```python
from build123d import *

# Parameters (mm, degrees)
SKETCH_1_W          = 99
SKETCH_1_H          = 40
EXTRUDE_1_DEPTH     = 4
SKETCH_2_R          = 2.025
CUT_EXTRUDE_1_DEPTH = 4
FILLET_1_R          = 3
CUT_EXTRUDE_2_DEPTH = 4
FILLET_2_R          = 1
SKETCH_4_R          = 7.5
CUT_EXTRUDE_3_DEPTH = 4
SKETCH_5_W          = 8
SKETCH_5_H          = 27
EXTRUDE_2_DEPTH     = 4
SKETCH_6_R          = 2.025
CUT_EXTRUDE_4_DEPTH = 4
FILLET_3_R          = 1


with BuildPart() as part:
    # 草图1 → 凸台-拉伸1 (new body)
    with BuildSketch(Plane(origin=(0, 0, 0), x_dir=(1, 0, 0), z_dir=(0, 1, 0))):
        Rectangle(SKETCH_1_W, SKETCH_1_H)
    extrude(amount=EXTRUDE_1_DEPTH)

    # 草图2 → 切除-拉伸1 (cut)
    with BuildSketch(Plane(origin=(0, 4, 0), x_dir=(1, 0, 0), z_dir=(0, 1, 0))):
        with Locations((-43.5, 15)):
            Circle(SKETCH_2_R)
        with Locations((-43.5, -15)):
            Circle(SKETCH_2_R)
        with Locations((-25.5, -15)):
            Circle(SKETCH_2_R)
        with Locations((-25.5, 15)):
            Circle(SKETCH_2_R)
    cut_extrude_1 = extrude(amount=-CUT_EXTRUDE_1_DEPTH, mode=Mode.SUBTRACT)

    # 镜向1: 切除-拉伸1 across plane
    add(cut_extrude_1.mirror(Plane(origin=(0, 0, 0), x_dir=(0, 0, 1), z_dir=(1, 0, 0))), mode=Mode.SUBTRACT)

    # 圆角1
    fillet_1_edges = [part.edges().sort_by_distance(p)[0] for p in [
        (49.5, 2, 20),
        (-49.5, 2, 20),
        (-49.5, 2, -20),
        (49.5, 2, -20),
    ]]
    fillet(fillet_1_edges, radius=FILLET_1_R)

    # 草图3 → 切除-拉伸2 (cut)
    with BuildSketch(Plane(origin=(0, 4, 0), x_dir=(1, 0, 0), z_dir=(0, 1, 0))):
        Polygon((-15.333333333, 13.5), (15.333333333, 13.5), (0, 2), align=None)
        Polygon((-21.5, 13.125), (-21.5, -13.125), (-4, 0), align=None)
        Polygon((-15.333333333, -13.5), (15.333333333, -13.5), (0, -2), align=None)
        Polygon((21.5, 13.125), (21.5, -13.125), (4, 0), align=None)
    extrude(amount=-CUT_EXTRUDE_2_DEPTH, mode=Mode.SUBTRACT)

    # 圆角2
    fillet_2_edges = [part.edges().sort_by_distance(p)[0] for p in [
        (15.333333333, 2, -13.5),
        (-15.333333333, 2, -13.5),
        (0, 2, -2),
        (15.333333333, 2, 13.5),
        (0, 2, 2),
        (-15.333333333, 2, 13.5),
        (-21.5, 2, 13.125),
        (-4, 2, 0),
        (-21.5, 2, -13.125),
        (21.5, 2, 13.125),
        (21.5, 2, -13.125),
        (4, 2, 0),
    ]]
    fillet(fillet_2_edges, radius=FILLET_2_R)

    # 草图4 → 切除-拉伸3 (cut)
    with BuildSketch(Plane(origin=(0, 4, 0), x_dir=(1, 0, 0), z_dir=(0, 1, 0))):
        with Locations((-34.5, 0)):
            Circle(SKETCH_4_R)
    cut_extrude_3 = extrude(amount=-CUT_EXTRUDE_3_DEPTH, mode=Mode.SUBTRACT)

    # 镜向2: 切除-拉伸3 across plane
    add(cut_extrude_3.mirror(Plane(origin=(0, 0, 0), x_dir=(0, 0, 1), z_dir=(1, 0, 0))), mode=Mode.SUBTRACT)

    # 草图5 → 凸台-拉伸2 (add)
    with BuildSketch(Plane(origin=(0, 4, 0), x_dir=(1, 0, 0), z_dir=(0, 1, 0))):
        Rectangle(SKETCH_5_W, SKETCH_5_H)
    extrude(amount=-EXTRUDE_2_DEPTH)

    # 草图6 → 切除-拉伸4 (cut)
    with BuildSketch(Plane(origin=(0, 4, 0), x_dir=(1, 0, 0), z_dir=(0, 1, 0))):
        with Locations((0, 5)):
            Circle(SKETCH_6_R)
        with Locations((0, -5)):
            Circle(SKETCH_6_R)
    extrude(amount=-CUT_EXTRUDE_4_DEPTH, mode=Mode.SUBTRACT)

    # 圆角3
    fillet_3_edges = [part.edges().sort_by_distance(p)[0] for p in [
        (-4, 2, 5),
        (4, 2, 5),
        (4, 2, -13.5),
        (-4, 2, 13.5),
        (-4, 2, -13.5),
        (-4, 2, -5),
        (4, 2, 13.5),
        (4, 2, -5),
    ]]
    fillet(fillet_3_edges, radius=FILLET_3_R)


solid = part.part
```
Can you work these out from the model? Positions are in its coordinate system, mm. Coordinates: 2 decimals unless noted, no trailing zeros. Loops run counter-clockwise (first coordinate to the right, second up) from the corner with the lowest first, then second, coordinate; pieces in that order, holes last.
1) Imagine slicing it at C-C on x = 34.5. List the corners of the cut face in (y, z) for me.
2) I need wall thicknesses on probe 1 along Z at (x, y) = (-43.5, 0.9) (3 decimals); probe 2 along X at (y, z) = (1.1, -15) (3 decimals); probe 3 along Z at (x, y) = (0, 1.6) (3 decimals). Which ranges of each line are inside material? Lowest first, please.
3) Imagine slicing it at B-B on z = -15. List the corners of the cut face in (x, y) for me (3 decimals).
4) For pin 1 (3.5 mm diameter, centred on x = 25.5, z = 15, fed in from +Y), with a flat end and sliding along its axis, tell me the tip position at first contact or that it passes through.
5) Thinking about a two-plate mould opening in X: for faces 1 (the flat face through (-1, 0, 0)), 2 (the flat face through (-4, 2, -10)), 3 (the cylindrical face through (48.6, 2.03, -19.14)), which applies, pulls with the +X half, pulls with the -X half, needs draft (parallel to the pull), parting line crosses it, or undercut?
6) Imagine slicing it at D-D on z = -5. List the corners of the cut face in (x, y) for me (3 decimals), plus the area to 3 significant figures.
7) Imagine slicing it at A-A on x = 0. List the corners of the cut face in (y, z) for me (3 decimals), plus the area to 3 significant figures.
Completed:
1. outline: (0, -20) - (4, -20) - (4, -7.5) - (0, -7.5) - close; (0, 7.5) - (4, 7.5) - (4, 20) - (0, 20) - close
2. probe 1: z = -20 to -17.025, -12.975 to 12.975, 17.025 to 20
2. probe 2: x = -49.5 to -45.525, -41.475 to -27.525, -23.475 to 23.475, 27.525 to 41.475, 45.525 to 49.5
2. probe 3: z = -20 to -7.025, -2.975 to 2.975, 7.025 to 20
3. outline: (-49.5, 0) - (-45.525, 0) - (-45.525, 4) - (-49.5, 4) - close; (-41.475, 0) - (-27.525, 0) - (-27.525, 4) - (-41.475, 4) - close; (-23.475, 0) - (23.475, 0) - (23.475, 4) - (-23.475, 4) - close; (27.525, 0) - (41.475, 0) - (41.475, 4) - (27.525, 4) - close; (45.525, 0) - (49.5, 0) - (49.5, 4) - (45.525, 4) - close
4. pin 1: passes through
5. face 1: needs draft
5. face 2: undercut
5. face 3: pulls with the +X half
6. outline: (-49.5, 0) - (-40.09, 0) - (-40.09, 4) - (-49.5, 4) - close; (-28.91, 0) - (-21.5, 0) - (-21.5, 4) - (-28.91, 4) - close; (-10.667, 0) - (-2.025, 0) - (-2.025, 4) - (-10.667, 4) - close; (2.025, 0) - (10.667, 0) - (10.667, 4) - (2.025, 4) - close; (21.5, 0) - (28.91, 0) - (28.91, 4) - (21.5, 4) - close; (40.09, 0) - (49.5, 0) - (49.5, 4) - (40.09, 4) - close
6. area: 204 mm2
7. outline: (0, -20) - (4, -20) - (4, -7.025) - (0, -7.025) - close; (0, -2.975) - (4, -2.975) - (4, 2.975) - (0, 2.975) - close; (0, 7.025) - (4, 7.025) - (4, 20) - (0, 20) - close
7. area: 128 mm2
